Design review of the part built by this model. Coordinates are the model's own, in mm. Round coordinates to 2 decimals unless told otherwise and drop trailing zeros. Loops run counter-clockwise (first coordinate to the right, second up) from the corner with the lowest first, then second, coordinate; pieces in that order, holes last. Notation, with made-up numbers: (77.5, 30) - (131.5, 30) arc R20 cw to (131.5, 36) - close; hole circle Ø6 at (-37, -6.75). An arc over 180 degrees is marked (long way). Return JSON: item names as keys, results as strings. Group by question number.
(1) Wall thickness on L1, parallel to X at y = 0.9, z = 65; L2, parallel to X at y = 0.6, z = 80; L3, parallel to Y at x = 2.5, z = 37: over which ranges is each line inside the solid? List them lowest first. Write a range as [from, to].
(2) Clearance check with flat-ended pins moving along their axes: pin 1 (2 mm diameter, centred on x = -1, z = 275, fed in from +Y); pin 2 (1.9 mm diameter, centred on x = 0, z = 35, fed in from +Y). State where each tip first meets the part, or that it passes through.
(3) We need section A-A, the plane z = 284. Write out the cut boundary in (x, y), and give its area (3 significant figures).
from build123d import *

# Parameters (mm, degrees)
EXTRUDE1_DEPTH             = 340
EXTRUDE2_REACH             = 342.052
SKETCH2_R                  = 1.2
SKETCH_R                   = 2.1
SKETCH_R_2                 = 1.2
EXTRUDE4_DEPTH             = 2.3
CHAMFER1_SIZE              = 0.2
LPATTERN1_COUNT            = 23
LPATTERN1_PITCH            = 15
CHAMFER1_OF_LPATTERN1_SIZE = 0.2


with BuildPart() as part:
    # Sketch1 → Extrude1 (new body)
    with BuildSketch(Plane.XY):
        with BuildLine():
            Line((-3.3, -2.4), (3.3, -2.4))
            Line((3.3, -2.4), (3.5, -2.2))
            Line((3.5, -2.2), (3.5, 0.106274607))
            ThreePointArc((3.5, 0.106274607), (3.091294745, 0.282570681), (2.840065792, 0.65))
            Line((2.840065792, 0.65), (2.340065792, 0.65))
            Line((2.340065792, 0.65), (2.340065792, 1.15))
            Line((2.340065792, 1.15), (2.840065792, 1.15))
            ThreePointArc((2.840065792, 1.15), (3.091294745, 1.517429319), (3.5, 1.693725393))
            Line((3.5, 1.693725393), (3.5, 2.2))
            Line((3.5, 2.2), (3.3, 2.4))
            Line((3.3, 2.4), (-3.3, 2.4))
            Line((-3.3, 2.4), (-3.5, 2.2))
            Line((-3.5, 2.2), (-3.5, 1.693725393))
            ThreePointArc((-3.5, 1.693725393), (-3.091294745, 1.517429319), (-2.840065792, 1.15))
            Line((-2.840065792, 1.15), (-2.340065792, 1.15))
            Line((-2.340065792, 1.15), (-2.340065792, 0.65))
            Line((-2.340065792, 0.65), (-2.840065792, 0.65))
            ThreePointArc((-2.840065792, 0.65), (-3.091294745, 0.282570681), (-3.5, 0.106274607))
            Line((-3.5, 0.106274607), (-3.5, -2.2))
            Line((-3.5, -2.2), (-3.3, -2.4))
        make_face()
    extrude(amount=EXTRUDE1_DEPTH)

    # Sketch2 → Extrude2 (cut, up to next)
    with BuildSketch(Plane(origin=(0, 2.4, 0), x_dir=(1, 0, 0), z_dir=(0, 1, 0)), mode=Mode.PRIVATE) as extrude2_sk1:
        with Locations(Location((0, -5, 0), (0, 0, 270))):
            Circle(SKETCH2_R)
    extrude2_tool1 = extrude(extrude2_sk1.sketch, amount=-EXTRUDE2_REACH, mode=Mode.PRIVATE) & part.part
    extrude2 = extrude2_tool1.solids().sort_by_distance((0, 2.4, 5))[0]
    add(extrude2, mode=Mode.SUBTRACT)

    # Sketch → Extrude4 (cut)
    with BuildSketch(Plane(origin=(0, 2.4, 0), x_dir=(1, 0, 0), z_dir=(0, 1, 0))):
        with Locations(Location((0, -5, 0), (0, 0, 270))):
            Circle(SKETCH_R)
        with Locations(Location((0, -5, 0), (0, 0, 270))):
            Circle(SKETCH_R_2, mode=Mode.SUBTRACT)
    extrude4 = extrude(amount=-EXTRUDE4_DEPTH, mode=Mode.SUBTRACT)

    # Chamfer1
    chamfer1_edges = [part.edges().sort_by_distance(p)[0] for p in [
        (0, -2.4, 3.8),
        (0, 2.4, 2.9),
    ]]
    chamfer(chamfer1_edges, length=CHAMFER1_SIZE)

    # LPattern1: Extrude2, Extrude4 ×23
    with Locations(*[(0, 0, i * LPATTERN1_PITCH) for i in range(1, LPATTERN1_COUNT)]):
        add(extrude2, mode=Mode.SUBTRACT)
        add(extrude4, mode=Mode.SUBTRACT)

    # Chamfer1 of LPattern1
    chamfer1_of_lpattern1_edges = [part.edges().sort_by_distance(p)[0] for p in [
        (0, -2.4, 18.8),
        (0, 2.4, 17.9),
        (0, -2.4, 33.8),
        (0, 2.4, 32.9),
        (0, -2.4, 48.8),
        (0, 2.4, 47.9),
        (0, -2.4, 63.8),
        (0, 2.4, 62.9),
        (0, -2.4, 78.8),
        (0, 2.4, 77.9),
        (0, -2.4, 93.8),
        (0, 2.4, 92.9),
        (0, -2.4, 108.8),
        (0, 2.4, 107.9),
        (0, -2.4, 123.8),
        (0, 2.4, 122.9),
        (0, -2.4, 138.8),
        (0, 2.4, 137.9),
        (0, -2.4, 153.8),
        (0, 2.4, 152.9),
        (0, -2.4, 168.8),
        (0, 2.4, 167.9),
        (0, -2.4, 183.8),
        (0, 2.4, 182.9),
        (0, -2.4, 198.8),
        (0, 2.4, 197.9),
        (0, -2.4, 213.8),
        (0, 2.4, 212.9),
        (0, -2.4, 228.8),
        (0, 2.4, 227.9),
        (0, -2.4, 243.8),
        (0, 2.4, 242.9),
        (0, -2.4, 258.8),
        (0, 2.4, 257.9),
        (0, -2.4, 273.8),
        (0, 2.4, 272.9),
        (0, -2.4, 288.8),
        (0, 2.4, 287.9),
        (0, -2.4, 303.8),
        (0, 2.4, 302.9),
        (0, -2.4, 318.8),
        (0, 2.4, 317.9),
        (0, -2.4, 333.8),
        (0, 2.4, 332.9),
    ]]
    chamfer(chamfer1_of_lpattern1_edges, length=CHAMFER1_OF_LPATTERN1_SIZE)


solid = part.part
Solutions:
{
 "1": {"L1": "[-2.34, -2.1], [2.1, 2.34]", "L2": "[-2.86, -2.1], [2.1, 2.86]", "L3": "[-2.4, 0.65], [1.15, 2.4]"},
 "2": {"pin 1": "y = 0.1", "pin 2": "through"},
 "3": {"outline": "(-3.5, -2.2) - (-3.3, -2.4) - (3.3, -2.4) - (3.5, -2.2) - (3.5, 0.11) arc R0.8 cw to (2.84, 0.65) - (2.34, 0.65) - (2.34, 1.15) - (2.84, 1.15) arc R0.8 cw to (3.5, 1.69) - (3.5, 2.2) - (3.3, 2.4) - (-3.3, 2.4) - (-3.5, 2.2) - (-3.5, 1.69) arc R0.8 cw to (-2.84, 1.15) - (-2.34, 1.15) - (-2.34, 0.65) - (-2.84, 0.65) arc R0.8 cw to (-3.5, 0.11) - close", "area": "31.4 mm^2"}
}
